```python
from build123d import *

# Parameters (mm, degrees)
F1_DEPTH = 4.54
F2_R     = 2.0625
F3_DEPTH = 10.16
F4_R     = 2.0625
F5_DEPTH = 10.16
F6_R     = 2.0625
F7_DEPTH = 10.16
F9_DEPTH = 9.081


with BuildPart() as f1:
    # F0 (on Top) → F1 (new body, symmetric)
    with BuildSketch(Plane.XY):
        Polygon((4.297212, 3.548719), (-4.297212, 3.548719), (-14.111018, 0.919118), (-12.93598, -3.466185), (-11.760941, -7.851489), (-4.54, -13.392312), (0, -13.392312), (4.54, -13.392312), (11.760941, -7.851489), (12.93598, -3.466185), (14.111018, 0.919118), align=None)
    extrude(amount=F1_DEPTH, both=True)

    # F2 (on face) → F3 (cut)
    with BuildSketch(Plane(origin=(-12.93598, -3.466185, 0), x_dir=(0.258819, -0.965926, 0), z_dir=(-0.965926, -0.258819, 0))):
        Circle(F2_R)
    extrude(amount=-F3_DEPTH, mode=Mode.SUBTRACT)

    # F4 (on face) → F5 (cut)
    with BuildSketch(Plane(origin=(12.93598, -3.466185, 0), x_dir=(0.258819, 0.965926, 0), z_dir=(0.965926, -0.258819, 0))):
        Circle(F4_R)
    extrude(amount=-F5_DEPTH, mode=Mode.SUBTRACT)

    # F6 (on face) → F7 (cut)
    with BuildSketch(Plane.XZ.offset(13.392312)):
        Circle(F6_R)
    extrude(amount=-F7_DEPTH, mode=Mode.SUBTRACT)

    # F8 (on face) → F9 (cut, through all)
    with BuildSketch(Plane.XY.offset(4.54)):
        Polygon((4.54, -13.392312), (11.760941, -7.851489), (4.54, -5.916643), align=None)
        Polygon((-11.760941, -7.851489), (-4.54, -13.392312), (-4.54, -5.916643), align=None)
    extrude(amount=-F9_DEPTH, mode=Mode.SUBTRACT)


solid = f1.part
```
Check sheet for the modelled part. Datum: model origin and axes. Units: mm. A direction names the side the tool comes from. Coordinates: 2 decimals unless noted, no trailing zeros. Loops run counter-clockwise (first coordinate to the right, second up) from the corner with the lowest first, then second, coordinate; pieces in that order, holes last.
1) Release check for a two-part mould opening along X. For faces 5 (the face through (0, -3, -4.54)), 6 (the face through (9.273, 2.216, 0.064)), 7 (the face through (0, -3.232, 0)), 8 (the face through (3.115, -0.864, 0.029)) record: released by +X, released by -X, zero draft, split by the parting line, or undercut.
2) Sectioned sample at D-D (z = 1). Record the boundary of the cut face in (x, y).
3) Sectioned sample at C-C (y = -11.5). Record the boundary of the cut face in (x, z) (1 decimal), and give its area (3 significant figures).
4) Access from +Z, -Z, +X, -X, +Y, -Y to the whole of each face (thin tool, end or side, straight path). Record for faces 1 (the face through (1.9, -8.4, -0.8)), 2 (the face through (-3.13, -0.81, 0.03)), 3 (the face through (4.54, -10, 0)), 4 (the face through (0, 3.549, 0)).
5) Gauge pin test, flat ends, axial feed: pin 1 (1 mm diameter, centred on y = -9, z = -3, fed in from +X); pin 2 (4 mm diameter, centred on x = -7, z = -1, fed in from +Y); pin 3 (2 mm diameter, centred on y = -8.5, z = -2, fed in from -X). Record the tip position at first contact, or that the pin passes through.
6) Sectioned sample at B-B (x = 0). Record the boundary of the cut face in (y, z), and give its area (3 significant figures).
7) Sectioned sample at A-A (z = -3). Record the boundary of the cut face in (x, y), and give its area (3 significant figures).
8) Material ranges on probe 1 along Z at (x, y) = (0, -6); probe 2 along X at (y, z) = (-10.5, 0.5); probe 3 along Y at (x, z) = (-9.75, 1), recorded low to high.
Check sheet entries:
1. face 5: zero draft
1. face 6: released by +X
1. face 7: undercut
1. face 8: undercut
2. outline: (-14.11, 0.92) - (-13.4, -1.72) - (-3.59, 0.91) - (-2.66, -2.58) - (-12.47, -5.21) - (-11.76, -7.85) - (-4.54, -5.92) - (-4.54, -13.39) - (-1.8, -13.39) - (-1.8, -3.23) - (1.8, -3.23) - (1.8, -13.39) - (4.54, -13.39) - (4.54, -5.92) - (11.76, -7.85) - (12.47, -5.21) - (2.66, -2.58) - (3.59, 0.91) - (13.4, -1.72) - (14.11, 0.92) - (4.3, 3.55) - (-4.3, 3.55) - close
3. outline: (-4.5, -4.5) - (4.5, -4.5) - (4.5, 4.5) - (-4.5, 4.5) - close; hole circle Ø4.1 at (0, 0)
3. area: 69.1 mm2
4. face 1: -Y
4. face 2: none
4. face 3: +Z, -Z, -Y
4. face 4: +Z, -Z, +X, -X, +Y
5. pin 1: stops at x = 4.54
5. pin 2: stops at y = 3.36
5. pin 3: stops at x = -11.86
6. outline: (-13.39, -4.54) - (3.55, -4.54) - (3.55, 4.54) - (-13.39, 4.54) - (-13.39, 2.06) - (-3.23, 2.06) - (-3.23, -2.06) - (-13.39, -2.06) - close
6. area: 112 mm2
7. outline: (-14.11, 0.92) - (-12.94, -3.47) - (-11.76, -7.85) - (-4.54, -5.92) - (-4.54, -13.39) - (4.54, -13.39) - (4.54, -5.92) - (11.76, -7.85) - (12.94, -3.47) - (14.11, 0.92) - (4.3, 3.55) - (-4.3, 3.55) - close
7. area: 312 mm2
8. probe 1: z = -4.54 to -2.06, 2.06 to 4.54
8. probe 2: x = -4.54 to -2, 2 to 4.54
8. probe 3: y = -7.31 to -4.48, -0.75 to 2.09
